Model file for the job. Use its own axes, mm. A direction names the side the tool comes from. Round coordinates to 2 decimals unless told otherwise and drop trailing zeros. Order: outer loops, then holes, each group sorted by start corner. A loop starts at its lowest first (then second) coordinate and runs counter-clockwise, first axis right, second up. Notation, with made-up numbers: (84, 46) -> (116, 46) arc R28 cw to (116, 77) -> close; hole circle Ø5 at (-26, -24). An arc over 180 degrees is marked (long way). Put each result on its own line as item: value. Start each with the question number.
Q1. Cut at D-D, the plane y = 6. List the corners of the cut face in (x, z).
Q2. Cut at B-B, the plane z = 10. List the corners of the cut face in (x, y) (3 decimals), and give its area (3 significant figures).
Q3. Cut at A-A, the plane x = 0. List the corners of the cut face in (y, z), and give its area (4 significant figures).
Q4. Flat gauge pins, fed straight in: P1, Ø4.5, axis at x = -20.14, y = 11.63, coming from the +Z side; P2, Ø1, axis at y = -10, z = 2.5, coming from the +X side; P3, Ø4, axis at x = -21, z = 15.5, coming from the -Y side; P4, Ø5, axis at x = -4, y = 11.5, coming from the -Z side. Where does each tip first touch, or does it go through?
Q5. Probe L1, parallel to Y at x = 0, z = 2.2; L2, parallel to X at y = -10.5, z = 16; L3, parallel to X at y = -13, z = 17. List the from-to ranges inside material, lowest first.
Q6. 3-axis set-ups, long thin cutter, end or side, ignore diameter. For faces 4 (the face through (-9.016, 20.25, 11.874)), 5 (the face through (18.387, -11.548, 15.084)), 6 (the face through (22.045, -2.317, 11.874)): which of +Z, -Z, +X, -X, +Y, -Y reach the whole face in a straight line?
Q7. Pull direction Y, two halves, no side cores. Call faces 1 (the face through (0, 20, 21)), 2 (the face through (0, 25, 15)), 3 (the face through (13.13, -18.07, 11.87)): released by +Y, released by -Y, zero draft, split by the parting line, or undercut.
Q8. Cut at C-C, the plane x = -12.5. List the corners of the cut face in (y, z).
from build123d import *

# Parameters (mm, degrees)
SKETCH2_W           = 3
SKETCH2_H           = 12
BOSS_EXTRUDE1_DEPTH = 18
CIRPATTERN1_COUNT   = 3
SKETCH4_R           = 1.75
CUT_EXTRUDE1_DEPTH  = 12
CIRPATTERN2_COUNT   = 3
SKETCH5_R           = 1.75
CUT_EXTRUDE2_DEPTH  = 44.819230938
CIRPATTERN3_COUNT   = 3


with BuildPart() as part:
    # Sketch2 → Revolve1 (revolve)
    with BuildSketch(Plane(origin=(0, 0, 0), x_dir=(0, 0, -1), z_dir=(1, 0, 0)), mode=Mode.PRIVATE) as revolve1_sk:
        with Locations((-1.5, 22.25)):
            Rectangle(SKETCH2_W, SKETCH2_H)
    revolve(revolve1_sk.sketch.rotate(Axis((0, 0, 0), (0, 0, 1)), 90), axis=Axis((0, 0, 0), (0, 0, 1)))

    # Sketch3 → Boss-Extrude1 (add)
    with BuildSketch(Plane.XY.offset(3)):
        with BuildLine():
            Line((-6.60947045, 14.845113687), (-11.490310167, 25.807659178))
            ThreePointArc((-11.490310167, 25.807659178), (0, 28.25), (11.490310167, 25.807659178))
            Line((11.490310167, 25.807659178), (6.60947045, 14.845113687))
            ThreePointArc((6.60947045, 14.845113687), (0, 16.25), (-6.60947045, 14.845113687))
        make_face()
    boss_extrude1 = extrude(amount=BOSS_EXTRUDE1_DEPTH)

    # CirPattern1: Boss-Extrude1 ×3 about axis
    cirpattern1_axis = Axis((0, 0, 0), (0, 0, 1))
    for i in range(1, CIRPATTERN1_COUNT):
        add(boss_extrude1.rotate(cirpattern1_axis, i * 360 / CIRPATTERN1_COUNT))

    # Sketch4 → Cut-Extrude1 (cut)
    with BuildSketch(Plane.XY.offset(21)):
        with Locations((0, 23.25)):
            Circle(SKETCH4_R)
    cut_extrude1 = extrude(amount=-CUT_EXTRUDE1_DEPTH, mode=Mode.SUBTRACT)

    # CirPattern2: Cut-Extrude1 ×3 about axis
    cirpattern2_axis = Axis((0, 0, 0), (0, 0, 1))
    for i in range(1, CIRPATTERN2_COUNT):
        add(cut_extrude1.rotate(cirpattern2_axis, i * 360 / CIRPATTERN2_COUNT), mode=Mode.SUBTRACT)

    # Sketch5 → Cut-Extrude2 (cut, through all)
    with BuildSketch(Plane.XY.offset(3)):
        with Locations((0, -23.25)):
            Circle(SKETCH5_R)
    cut_extrude2 = extrude(amount=-CUT_EXTRUDE2_DEPTH, mode=Mode.SUBTRACT)

    # CirPattern3: Cut-Extrude2 ×3 about axis
    cirpattern3_axis = Axis((0, 0, 0), (0, 0, 1))
    for i in range(1, CIRPATTERN3_COUNT):
        add(cut_extrude2.rotate(cirpattern3_axis, i * 360 / CIRPATTERN3_COUNT), mode=Mode.SUBTRACT)


solid = part.part
Ans:
1. outline: (-27.61, 0) -> (-15.1, 0) -> (-15.1, 3) -> (-27.61, 3) -> close; (15.1, 0) -> (27.61, 0) -> (27.61, 3) -> (15.1, 3) -> close
2. outline: (-28.095, -2.953) arc R28.25 ccw to (-16.605, -22.855) -> (-9.552, -13.147) arc R16.25 cw to (-16.161, -1.699) -> close; (-11.49, 25.808) -> (-6.609, 14.845) arc R16.25 cw to (6.609, 14.845) -> (11.49, 25.808) arc R28.25 ccw to start; (9.552, -13.147) -> (16.605, -22.855) arc R28.25 ccw to (28.095, -2.953) -> (16.161, -1.699) arc R16.25 cw to start; hole circle Ø3.5 at (-20.135, -11.625); hole circle Ø3.5 at (0, 23.25); hole circle Ø3.5 at (20.135, -11.625)
2. area: 642 mm^2
3. outline: (-28.25, 0) -> (-25, 0) -> (-25, 3) -> (-28.25, 3) -> close; (-21.5, 0) -> (-16.25, 0) -> (-16.25, 3) -> (-21.5, 3) -> close; (16.25, 0) -> (28.25, 0) -> (28.25, 21) -> (25, 21) -> (25, 9) -> (21.5, 9) -> (21.5, 21) -> (16.25, 21) -> close
3. area: 235.5 mm^2
4. P1: stops at z = 3
4. P2: stops at x = 26.6
4. P3: stops at y = -20.91
4. P4: passes through
5. L1: y = -28.25 to -25, -21.5 to -16.25, 16.25 to 28.25
5. L2: x = -26.23 to -21.48, -18.79 to -12.4, 12.4 to 18.79, 21.48 to 26.23
5. L3: x = -25.08 to -21.22, -19.05 to -9.75, 9.75 to 19.05, 21.22 to 25.08
6. face 4: +Z, -X
6. face 5: +Z
6. face 6: +Z, +X, +Y
7. face 1: zero draft
7. face 2: undercut
7. face 3: released by -Y
8. outline: (-25.33, 0) -> (-10.38, 0) -> (-10.38, 21) -> (-17.2, 21) -> (-17.2, 3) -> (-25.33, 3) -> close; (10.38, 0) -> (25.33, 0) -> (25.33, 3) -> (10.38, 3) -> close
